```python
from build123d import *

# Parameters (mm, degrees)
CROQUIS1_W              = 20.5
CROQUIS1_H              = 20.5
SALIENTE_EXTRUIR1_DEPTH = 7
REDONDEO1_R             = 3
CROQUIS2_R              = 6.35
SALIENTE_EXTRUIR2_DEPTH = 2.7
CROQUIS3_R              = 3.15
CORTAR_EXTRUIR1_DEPTH   = 10.7
CROQUIS4_R              = 1.35
CORTAR_EXTRUIR2_DEPTH   = 8
CORTAR_EXTRUIR3_REACH   = 22.5
CROQUIS5_R              = 2.5


with BuildPart() as part:
    # Croquis1 → Saliente-Extruir1 (new body)
    with BuildSketch(Plane.XY):
        Rectangle(CROQUIS1_W, CROQUIS1_H)
    extrude(amount=SALIENTE_EXTRUIR1_DEPTH)

    # Redondeo1
    redondeo1_edges = [part.edges().sort_by_distance(p)[0] for p in [
        (10.25, -10.25, 3.5),
        (-10.25, -10.25, 3.5),
        (-10.25, 10.25, 3.5),
        (10.25, 10.25, 3.5),
    ]]
    fillet(redondeo1_edges, radius=REDONDEO1_R)

    # Croquis2 → Saliente-Extruir2 (add)
    with BuildSketch(Plane.XY.offset(7)):
        Circle(CROQUIS2_R)
    extrude(amount=SALIENTE_EXTRUIR2_DEPTH)

    # Croquis3 → Cortar-Extruir1 (cut, through all)
    with BuildSketch(Plane.XY.offset(9.7)):
        Circle(CROQUIS3_R)
    extrude(amount=-CORTAR_EXTRUIR1_DEPTH, mode=Mode.SUBTRACT)

    # Croquis4 → Cortar-Extruir2 (cut, through all)
    with BuildSketch(Plane.XY.offset(7)):
        with Locations((-6.91550432, 6.91550432)):
            Circle(CROQUIS4_R)
        with Locations((6.91550432, 6.91550432)):
            Circle(CROQUIS4_R)
        with Locations((6.91550432, -6.91550432)):
            Circle(CROQUIS4_R)
        with Locations((-6.91550432, -6.91550432)):
            Circle(CROQUIS4_R)
    extrude(amount=-CORTAR_EXTRUIR2_DEPTH, mode=Mode.SUBTRACT)

    # Croquis5 → Cortar-Extruir3 (cut, up to next)
    with BuildSketch(Plane(origin=(0, 10.25, 0), x_dir=(1, 0, 0), z_dir=(0, 1, 0)), mode=Mode.PRIVATE) as cortar_extruir3_sk1:
        with Locations((0, -3.5)):
            Circle(CROQUIS5_R)
    cortar_extruir3_tool1 = extrude(cortar_extruir3_sk1.sketch, amount=-CORTAR_EXTRUIR3_REACH, mode=Mode.PRIVATE) & part.part
    add(cortar_extruir3_tool1.solids().sort_by_distance((0, 10.25, 3.5))[0], mode=Mode.SUBTRACT)


solid = part.part
```
CAD build for the part. Positions are in the model's coordinates, mm. A direction names the side the tool comes from. Give positions to 0.01 mm unless a question says otherwise; leave off trailing zeros. Order: outer loops, then holes, each group sorted by start corner. A loop starts at its lowest first (then second) coordinate and runs counter-clockwise, first axis right, second up. Notation, with made-up numbers: M -17,82.5 L 33,82.5 A18 cw 33,88.5 Z; hole C 57.5,-28.75 d10. An arc over 180 degrees is marked long. Put each result on its own line as item: value. Start each with the question number.
(1) Drill centre lines: line 1 along X through (y, z) = (4, 3.5); line 2 along Z through (x, y) = (-4.75, -4.75); line 3 along Y through (x, z) = (2.75, 6.5). Where is each one in solid material? Low to high.
(2) Flat gauge pins, fed straight in: pin 1 Ø2 at (x, y) = (-6.92, 6.92) entering from -Z; pin 2 Ø4 at (x, y) = (7.5, -4.5) entering from +Z. Where does each tip first touch, or does it go through?
(3) Saw through at C-C, the plane z = 2.5. Write the cut outline in (x, y).
(4) Saw through at A-A, the plane x = 0. Write the cut outline in (y, z), then the cut area to 3 significant figures.
(5) Which spindle directions (+Z, -Z, +X, -X, +Y, -Y) get a long thin tool onto all of the face, cutting with end or side? Do faces 1 (the cylindrical face through (2.385, 6.141, 2.749)), 2 (the flat face through (-5, 5, 7)), 3 (the cylindrical face through (-0.683, -3.075, 4.918)). Say none if no direction does.
(6) Saw through at B-B, the plane y = 0. Write the cut outline in (x, z).
(7) Mould opens along Y. For faces 4 (the cylindrical face through (-7.91, 7.83, 3.55)), 5 (the flat face through (0, -10.25, 3)), 6 (the flat face through (-2, 3, 9.7)), 7 (the cylindrical face through (-7.91, -6, 3.55)) say: +Y half, -Y half, draft (parallel to the pull), parting line (faces both ways), or undercut.
(8) Saw through at D-D, the plane z = 7.5. Write the cut outline in (x, y).
Check result:
1. line 1: x = -10.25 to -2.5, 2.5 to 10.25
1. line 2: z = 0 to 7
1. line 3: y = -10.25 to -1.54, 1.54 to 10.25
2. pin 1: passes through
2. pin 2: stops at z = 7
3. outline: M -10.25,-7.25 A3 ccw -7.25,-10.25 L 7.25,-10.25 A3 ccw 10.25,-7.25 L 10.25,7.25 A3 ccw 7.25,10.25 L 2.29,10.25 L 2.29,2.16 A3.15 cw long -2.29,2.16 L -2.29,10.25 L -7.25,10.25 A3 ccw -10.25,7.25 Z; hole C -6.92,-6.92 d2.7; hole C -6.92,6.92 d2.7; hole C 6.92,-6.92 d2.7; hole C 6.92,6.92 d2.7
4. outline: M -10.25,0 L -3.15,0 L -3.15,9.7 L -6.35,9.7 L -6.35,7 L -10.25,7 Z; M 3.15,0 L 10.25,0 L 10.25,1 L 3.15,1 Z; M 3.15,6 L 10.25,6 L 10.25,7 L 6.35,7 L 6.35,9.7 L 3.15,9.7 Z
4. area: 81.2 mm2
5. face 1: +Y
5. face 2: +Z
5. face 3: +Z, -Z
6. outline: M -10.25,0 L -3.15,0 L -3.15,9.7 L -6.35,9.7 L -6.35,7 L -10.25,7 Z; M 3.15,0 L 10.25,0 L 10.25,7 L 6.35,7 L 6.35,9.7 L 3.15,9.7 Z
7. face 4: undercut
7. face 5: -Y half
7. face 6: draft
7. face 7: undercut
8. outline: C 0,0 d12.7; hole C 0,0 d6.3
